from build123d import *

# Parameters (mm, degrees)
SKETCH1_W                    = 80
SKETCH1_H                    = 40
SKETCH1_R                    = 10
BOSS_EXTRUDE1_DEPTH          = 3
SKETCH2_W                    = 80
SKETCH2_H                    = 4.5
BOSS_EXTRUDE2_DEPTH          = 9
SKETCH3_W                    = 2.8
SKETCH3_H                    = 7
SKETCH3_W_2                  = 2.5
SKETCH3_H_2                  = 6.8
CUT_EXTRUDE1_DEPTH           = 80
SKETCH5_R                    = 1.75
CUT_EXTRUDE3_DEPTH           = 1
SKETCH4_R                    = 3.75
CUT_EXTRUDE4_DEPTH           = 2
CUT_EXTRUDE4_DRAFT           = -45
CUT_EXTRUDE4_PROFILE_2_DEPTH = 2
CUT_EXTRUDE4_PROFILE_2_DRAFT = -45
CUT_EXTRUDE4_PROFILE_3_DEPTH = 2
CUT_EXTRUDE4_PROFILE_3_DRAFT = -45
CUT_EXTRUDE4_PROFILE_4_DEPTH = 2
CUT_EXTRUDE4_PROFILE_4_DRAFT = -45
FILLET1_R                    = 7
SKETCH6_W                    = 27
SKETCH6_H                    = 6
BOSS_EXTRUDE3_DEPTH          = 7
SKETCH7_R                    = 3
BOSS_EXTRUDE4_DEPTH          = 2


with BuildPart() as part:
    # Sketch1 → Boss-Extrude1 (new body)
    with BuildSketch(Plane(origin=(0, 0, 0), x_dir=(1, 0, 0), z_dir=(0, 1, 0))):
        Rectangle(SKETCH1_W, SKETCH1_H)
        with Locations(Location((0, 0, 0), (0, 0, 270))):
            Circle(SKETCH1_R, mode=Mode.SUBTRACT)
    extrude(amount=BOSS_EXTRUDE1_DEPTH)

    # Sketch2 → Boss-Extrude2 (add)
    with BuildSketch(Plane(origin=(0, 3, 0), x_dir=(1, 0, 0), z_dir=(0, 1, 0))):
        with Locations((0, 17.75)):
            Rectangle(SKETCH2_W, SKETCH2_H)
        with Locations((0, -17.75)):
            Rectangle(SKETCH2_W, SKETCH2_H)
    extrude(amount=BOSS_EXTRUDE2_DEPTH)

    # Sketch3 → Cut-Extrude1 (cut)
    with BuildSketch(Plane.ZY.offset(40)):
        with Locations((-16.9, 6.5)):
            Rectangle(SKETCH3_W, SKETCH3_H)
        with Locations((16.75, 6.4)):
            Rectangle(SKETCH3_W_2, SKETCH3_H_2)
    extrude(amount=-CUT_EXTRUDE1_DEPTH, mode=Mode.SUBTRACT)

    # Sketch5 → Cut-Extrude3 (cut)
    with BuildSketch(Plane.XZ):
        with Locations(Location((-15.5, 8, 0), (0, 0, 270))):
            Circle(SKETCH5_R)
        with Locations(Location((-15.5, -8, 0), (0, 0, 270))):
            Circle(SKETCH5_R)
        with Locations(Location((15.5, 8, 0), (0, 0, 270))):
            Circle(SKETCH5_R)
        with Locations(Location((15.5, -8, 0), (0, 0, 270))):
            Circle(SKETCH5_R)
    extrude(amount=-CUT_EXTRUDE3_DEPTH, mode=Mode.SUBTRACT)


with BuildPart() as cut_extrude4_tool:
    # Sketch4 → Cut-Extrude4 (with draft: the straight prism first)
    with BuildSketch(Plane(origin=(0, 3, 0), x_dir=(1, 0, 0), z_dir=(0, 1, 0))):
        with Locations((-15.5, 8)):
            Circle(SKETCH4_R)
    extrude(amount=-CUT_EXTRUDE4_DEPTH)
    # Cut-Extrude4: the draft: its side faces are tilted about the plane it starts from
    cut_extrude4_sides = [cut_extrude4_tool.faces().sort_by_distance(p)[0] for p in [
        (-19.25, 2, -8),
    ]]
    draft(cut_extrude4_sides, Plane(origin=(0, 3, 0), x_dir=(1, 0, 0), z_dir=(0, 1, 0)), CUT_EXTRUDE4_DRAFT)


with BuildPart() as part_1:
    add(part.part)

    # Cut-Extrude4: cut by cut_extrude4_tool
    add(cut_extrude4_tool.part, mode=Mode.SUBTRACT)


with BuildPart() as cut_extrude4_profile_2_tool:
    # Sketch4 → Cut-Extrude4 profile 2 (with draft: the straight prism first)
    with BuildSketch(Plane(origin=(0, 3, 0), x_dir=(1, 0, 0), z_dir=(0, 1, 0))):
        with Locations((-15.5, -8)):
            Circle(SKETCH4_R)
    extrude(amount=-CUT_EXTRUDE4_PROFILE_2_DEPTH)
    # Cut-Extrude4 profile 2: the draft: its side faces are tilted about the plane it starts from
    cut_extrude4_profile_2_sides = [cut_extrude4_profile_2_tool.faces().sort_by_distance(p)[0] for p in [
        (-19.25, 2, 8),
    ]]
    draft(cut_extrude4_profile_2_sides, Plane(origin=(0, 3, 0), x_dir=(1, 0, 0), z_dir=(0, 1, 0)), CUT_EXTRUDE4_PROFILE_2_DRAFT)


with BuildPart() as part_2:
    add(part_1.part)

    # Cut-Extrude4 profile 2: cut by cut_extrude4_profile_2_tool
    add(cut_extrude4_profile_2_tool.part, mode=Mode.SUBTRACT)


with BuildPart() as cut_extrude4_profile_3_tool:
    # Sketch4 → Cut-Extrude4 profile 3 (with draft: the straight prism first)
    with BuildSketch(Plane(origin=(0, 3, 0), x_dir=(1, 0, 0), z_dir=(0, 1, 0))):
        with Locations((15.5, -8)):
            Circle(SKETCH4_R)
    extrude(amount=-CUT_EXTRUDE4_PROFILE_3_DEPTH)
    # Cut-Extrude4 profile 3: the draft: its side faces are tilted about the plane it starts from
    cut_extrude4_profile_3_sides = [cut_extrude4_profile_3_tool.faces().sort_by_distance(p)[0] for p in [
        (11.75, 2, 8),
    ]]
    draft(cut_extrude4_profile_3_sides, Plane(origin=(0, 3, 0), x_dir=(1, 0, 0), z_dir=(0, 1, 0)), CUT_EXTRUDE4_PROFILE_3_DRAFT)


with BuildPart() as part_3:
    add(part_2.part)

    # Cut-Extrude4 profile 3: cut by cut_extrude4_profile_3_tool
    add(cut_extrude4_profile_3_tool.part, mode=Mode.SUBTRACT)


with BuildPart() as cut_extrude4_profile_4_tool:
    # Sketch4 → Cut-Extrude4 profile 4 (with draft: the straight prism first)
    with BuildSketch(Plane(origin=(0, 3, 0), x_dir=(1, 0, 0), z_dir=(0, 1, 0))):
        with Locations((15.5, 8)):
            Circle(SKETCH4_R)
    extrude(amount=-CUT_EXTRUDE4_PROFILE_4_DEPTH)
    # Cut-Extrude4 profile 4: the draft: its side faces are tilted about the plane it starts from
    cut_extrude4_profile_4_sides = [cut_extrude4_profile_4_tool.faces().sort_by_distance(p)[0] for p in [
        (11.75, 2, -8),
    ]]
    draft(cut_extrude4_profile_4_sides, Plane(origin=(0, 3, 0), x_dir=(1, 0, 0), z_dir=(0, 1, 0)), CUT_EXTRUDE4_PROFILE_4_DRAFT)


with BuildPart() as part_4:
    add(part_3.part)

    # Cut-Extrude4 profile 4: cut by cut_extrude4_profile_4_tool
    add(cut_extrude4_profile_4_tool.part, mode=Mode.SUBTRACT)

    # Fillet1
    fillet1_edges = [part_4.edges().sort_by_distance(p)[0] for p in [
        (40, 6, 20),
        (40, 6, -20),
        (-40, 6, 20),
        (-40, 6, -20),
    ]]
    fillet(fillet1_edges, radius=FILLET1_R)

    # Sketch6 → Boss-Extrude3 (add)
    with BuildSketch(Plane(origin=(0, 3, 0), x_dir=(1, 0, 0), z_dir=(0, 1, 0))):
        with Locations((-26.5, 0.145287111)):
            Rectangle(SKETCH6_W, SKETCH6_H)
        with Locations((26.5, 0.145287111)):
            Rectangle(SKETCH6_W, SKETCH6_H)
    extrude(amount=BOSS_EXTRUDE3_DEPTH)

    # Sketch7 → Boss-Extrude4 (add)
    with BuildSketch(Plane(origin=(0, 10, 0), x_dir=(1, 0, 0), z_dir=(0, 1, 0))):
        with BuildLine():
            Line((40, 6), (18.672144385, 6))
            ThreePointArc((18.672144385, 6), (15.5, 4.25), (12.327855615, 6))
            Line((12.327855615, 6), (-12.327855615, 6))
            ThreePointArc((-12.327855615, 6), (-15.5, 4.25), (-18.672144385, 6))
            Line((-18.672144385, 6), (-40, 6))
            Line((-40, 6), (-40, -6))
            Line((-40, -6), (-18.672144385, -6))
            ThreePointArc((-18.672144385, -6), (-15.5, -4.25), (-12.327855615, -6))
            Line((-12.327855615, -6), (12.327855615, -6))
            ThreePointArc((12.327855615, -6), (15.5, -4.25), (18.672144385, -6))
            Line((18.672144385, -6), (40, -6))
            Line((40, -6), (40, 6))
        make_face()
        with Locations(Location((0, 0, 0), (0, 0, 270))):
            Circle(SKETCH7_R, mode=Mode.SUBTRACT)
    extrude(amount=BOSS_EXTRUDE4_DEPTH)


solid = part_4.part
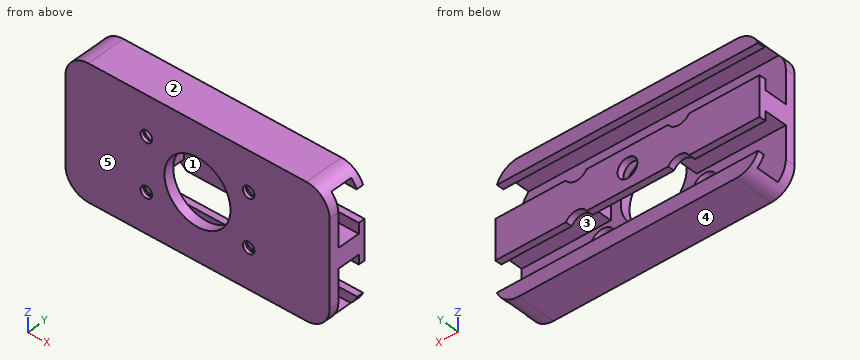
Design review of the part built by this model. Coordinates are the model's own, in mm. Face numbers are marked on the shaded views. A direction names the side the tool comes from. Coordinates: 2 decimals unless noted, no trailing zeros. Loops run counter-clockwise (first coordinate to the right, second up) from the corner with the lowest first, then second, coordinate; pieces in that order, holes last. Notation, with made-up numbers: M -36,-9 L 1,-9 A25 cw 1,22 Z; hole C 18,68 d5. An arc over 180 degrees is marked long. Answer as CSV lines item,"result".
Item 1: Add section C-C on y = 8.5. State the section outline as (x, z) points, plus the area to 3 significant figures.
Answer list:
outline,"M -40,-3.15 L -13,-3.15 L -13,2.85 L -40,2.85 Z; M -37.9,18 L 37.9,18 A7 ccw 33,20 L -33,20 A7 ccw Z; M -37.57,-18.3 A7 ccw -33,-20 L 33,-20 A7 ccw 37.57,-18.3 Z; M 13,-3.15 L 40,-3.15 L 40,2.85 L 13,2.85 Z"
area,"592 mm²"
Item 2: For P1, Ø3, axis at x = -15.5, z = -8, coming from the +Y side, flat-tipped, find the tip position at first contact; note if it passes through.
Answer list:
P1,"through"
Item 3: The part is to be moulded in two halves that separate along Y. For the marked faces 3, 4 and 5, say which applies: pulls with the +Y half, pulls with the -Y half, needs draft (parallel to the pull), parting line crosses it, or undercut.
Answer list:
face 3,"undercut"
face 4,"needs draft"
face 5,"pulls with the -Y half"
Item 4: Machinability: for the marked faces 1 and 2, which of the approach directions +Z, -Z, +X, -X, +Y, -Y give a long, thin tool a straight path to every point of the face, cutting with its end or side? Answer none if there is none.
Answer list:
face 1,"none"
face 2,"+Z, +X, -X, +Y, -Y"
Item 5: Add section A-A on z = 8. State the section outline as (x, y) points, plus the area to 3 significant figures.
Answer list:
outline,"M -40,0 L -17.25,0 L -17.25,1 L -19.25,3 L -40,3 Z; M -13.75,0 L -6,0 L -6,3 L -11.75,3 L -13.75,1 Z; M 6,0 L 13.75,0 L 13.75,1 L 11.75,3 L 6,3 Z; M 17.25,0 L 40,0 L 40,3 L 19.25,3 L 17.25,1 Z"
area,"175 mm²"
Item 6: Add section B-B on x = 15.5. Count the separate pieces of the cut face and the enclosed holes in it, plus the area to 3 significant figures.
Answer list:
separate pieces,"3"
enclosed holes,"0"
area,"194 mm²"
Item 7: For probe 1 along X at (y, z) = (0.3, 8); probe 2 along Z at (x, y) = (21, 5); probe 3 along Z at (x, y) = (-15.5, 0.65), list the stretches that pass through material, from the lowest coordinate up.
Answer list:
probe 1,"-40 to -17.25, -13.75 to -6, 6 to 13.75, 17.25 to 40"
probe 2,"-20 to -18.3, -3.15 to 2.85, 18 to 20"
probe 3,"-20 to -9.75, -6.25 to 6.25, 9.75 to 20"
Item 8: Add section D-D on z = 0. State the section outline as (x, y) points, plus the area to 3 significant figures.
Answer list:
outline,"M -40,0 L -10,0 L -10,3 L -13,3 L -13,10 L -3,10 L -3,12 L -40,12 Z; M 3,10 L 13,10 L 13,3 L 10,3 L 10,0 L 40,0 L 40,12 L 3,12 Z"
area,"706 mm²"
